```python
from build123d import *

# Parameters (mm, degrees)
F0_W     = 41
F0_H     = 11
F1_DEPTH = 2
F0_W_2   = 8
F0_H_2   = 3
F2_DEPTH = 3.5
F3_W     = 3.5
F3_H     = 2
F4_DEPTH = 3
F5_W     = 3.5
F5_H     = 2
F6_DEPTH = 3


with BuildPart() as f1:
    # F0 (on Top) → F1 (new body)
    with BuildSketch(Plane.XY):
        with Locations((-20.5, -5.5)):
            Rectangle(F0_W, F0_H)
        Polygon((-39, -9), (-39, -2), (-29, -2), (-29, -4), (-29, -7), (-29, -9), align=None, mode=Mode.SUBTRACT)
        Polygon((-2, -9), (-12, -9), (-12, -7), (-12, -4), (-12, -2), (-2, -2), align=None, mode=Mode.SUBTRACT)
    extrude(amount=F1_DEPTH)

    # F0 (on Top) → F2 (join)
    with BuildSketch(Plane.XY):
        with Locations((-33, -5.5)):
            Rectangle(F0_W_2, F0_H_2)
        with Locations((-8, -5.5)):
            Rectangle(F0_W_2, F0_H_2)
    extrude(amount=F2_DEPTH)

    # F3 (on face) → F4 (cut, through all)
    with BuildSketch(Plane.XZ.offset(7)):
        Polygon((-33, 3.5), (-29, 2), (-29, 3.5), align=None)
        with Locations((-33, 1)):
            Rectangle(F3_W, F3_H)
    extrude(amount=-F4_DEPTH, mode=Mode.SUBTRACT)

    # F5 (on face) → F6 (cut, through all)
    with BuildSketch(Plane.XZ.offset(7)):
        Polygon((-8, 3.5), (-12, 3.5), (-12, 2), align=None)
        with Locations((-8, 1)):
            Rectangle(F5_W, F5_H)
    extrude(amount=-F6_DEPTH, mode=Mode.SUBTRACT)


solid = f1.part
```
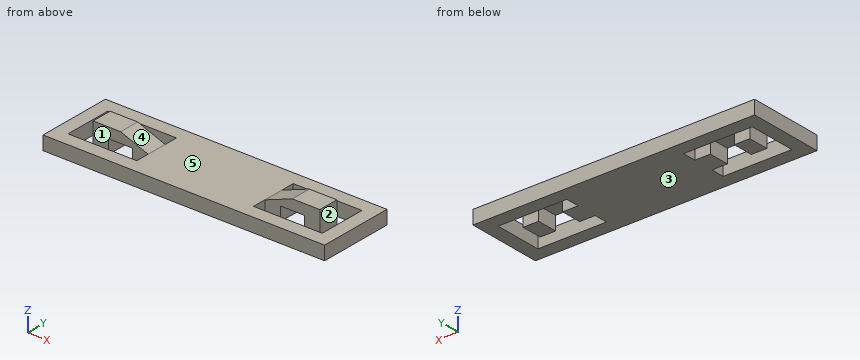
Here's how the part is built. I have some questions about the finished solid (model axes, mm). Face numbers are marked on the shaded views. A direction names the side the tool comes from. Give positions to 0.01 mm unless a question says otherwise; leave off trailing zeros. Write each loop counter-clockwise with the first axis right and the second up, starting at its lowest first coordinate (ties: lowest second). Pieces come first, ordered by that corner, then holes. Notation, with made-up numbers: M 68,-7.75 L 102,-7.75 A26 ccw 102,12.25 Z; hole C 0,55 d9. An arc over 180 degrees is marked long. Put each result on its own line as item: value. Start each with the question number.
Item 1: If we section it at B-B, the plane y = -3.25: Write out the boundary of the cut face in (x, z), then the cut area to 3 significant figures.
Item 2: Will this pin go through, and if not, where does the flat tip stop? pin 1 (3 mm diameter, centred on x = -6, y = -3, fed in from -Z).
Item 3: On a 3-axis mill with a long thin cutter (end or side, diameter ignored), from which of +Z, -Z, +X, -X, +Y, -Y can I reach the whole of each face in a straight line? I mean the marked faces 4 and 5. Say none if no direction works.
Item 4: If we section it at C-C, the plane x = -32: Write out the boundary of the cut face in (y, z) (3 decimals).
Item 5: Thinking about a two-plate mould opening in X: for the marked faces 1, 2 and 3, which applies, +X half, -X half, draft (parallel to the pull), parting line (faces both ways), or undercut?
Item 6: I need wall thicknesses on L1, parallel to Y at x = -35.5, z = 0.45; L2, parallel to X at y = -2.75, z = 1.95; L3, parallel to Y at x = -3, z = 1.25. Which ranges of each line are inside material? Lowest first, please. Write a range as from..to.
Item 7: If we section it at D-D, the plane z = 3.1: Write out the boundary of the cut face in (x, y).
Item 8: If we section it at A-A, the plane z = 1.35: Write out the boundary of the cut face in (x, y).
Values:
1. outline: M -41,0 L -39,0 L -39,2 L -41,2 Z; M -29,0 L -12,0 L -12,2 L -29,2 Z; M -2,0 L 0,0 L 0,2 L -2,2 Z
1. area: 42.0 mm²
2. pin 1: z = 0
3. face 4: +Z, +Y, -Y
3. face 5: +Z
4. outline: M -11,0 L -9,0 L -9,2 L -11,2 Z; M -7,2 L -4,2 L -4,3.125 L -7,3.125 Z; M -2,0 L 0,0 L 0,2 L -2,2 Z
5. face 1: undercut
5. face 2: undercut
5. face 3: draft
6. L1: -11..-9, -7..-4, -2..0
6. L2: -41..-39, -29..-12, -2..0
6. L3: -11..-9, -2..0
7. outline: M -37,-7 L -31.93,-7 L -31.93,-4 L -37,-4 Z; M -9.07,-7 L -4,-7 L -4,-4 L -9.07,-4 Z
8. outline: M -41,-11 L 0,-11 L 0,0 L -41,0 Z; M -37,-7 L -34.75,-7 L -34.75,-4 L -37,-4 Z; M -6.25,-7 L -4,-7 L -4,-4 L -6.25,-4 Z; hole M -39,-9 L -29,-9 L -29,-7 L -31.25,-7 L -31.25,-4 L -29,-4 L -29,-2 L -39,-2 Z; hole M -12,-9 L -2,-9 L -2,-2 L -12,-2 L -12,-4 L -9.75,-4 L -9.75,-7 L -12,-7 Z
